Here's how the part is built. I have some questions about the finished solid (model axes, mm). A direction names the side the tool comes from. Coordinates: 2 decimals unless noted, no trailing zeros. Loops run counter-clockwise (first coordinate to the right, second up) from the corner with the lowest first, then second, coordinate; pieces in that order, holes last. Notation, with made-up numbers: (39.25, -2) -> (83.25, -2) arc R22 cw to (83.25, 24) -> close; hole circle Ø9 at (85, 62). An arc over 180 degrees is marked (long way). Answer as a JSON object with one key per item and string values. Group by question number.
1) I want a section at C-C (z = 0.9). Write out the boundary of the cut face in (x, y) (3 decimals).
2) I want a section at B-B (y = 8). Write out the boundary of the cut face in (x, z).
3) If we mould it in two halves opening along X, with no side actions, what happens to faces 6 (the flat face through (0, -33, 1)), 7 (the cylindrical face through (18.402, -32.257, 1.479)), 8 (the flat face through (0, -30, 1))? For each: +X half, -X half, draft (parallel to the pull), parting line (faces both ways), or undercut.
4) I want a section at D-D (x = 24.5). Write out the boundary of the cut face in (y, z) (3 decimals).
5) I want a section at A-A (x = 5.5). Write out the boundary of the cut face in (y, z) (3 decimals), then the cut area to 3 significant figures.
6) I need wall thicknesses on probe 1 along Y at (x, z) = (5.5, 1.8) (3 decimals); probe 2 along Y at (x, z) = (-0.5, 1.9); probe 3 along X at (y, z) = (13, 0.8). Which ranges of each line are inside material? Lowest first, please. Write a range as [from, to].
7) I'm going to push flat-ended pins straight in: pin 1 (1.5 mm diameter, centred on x = -15.5, z = 1.5, fed in from +Y); pin 2 (0.9 mm diameter, centred on x = 13.5, z = 1.5, fed in from -Y); pin 3 (1.5 mm diameter, centred on y = 19.5, z = 1, fed in from -X). Where does each tip first touch, or does it pass through?
8) Which directions (+Z, -Z, +X, -X, +Y, -Y) give clear straight access to the entire face, cutting with the end or side of a thin tool? Please do faces 1 (the flat face through (-14, -30, 1)), 2 (the flat face through (-16, -8.425, 1)), 3 (the cylindrical face through (-18.6, -32.2, 1.5)), 4 (the flat face through (0, 33, 1)), 5 (the flat face through (16, -27, 1)).
```python
from build123d import *

# Parameters (mm, degrees)
SALIENTE_EXTRUIR1_DEPTH = 3


with BuildPart() as part:
    # Croquis1 → Saliente-Extruir1 (new body)
    with BuildSketch(Plane.XY):
        with BuildLine():
            Line((-13, -33), (13, -33))
            ThreePointArc((13, -33), (18.477225575, -32.235384062), (23.535653753, -30))
            Line((23.535653753, -30), (4.502856857, -30))
            Line((4.502856857, -30), (4.502856857, -27))
            Line((4.502856857, -27), (27.282856857, -27))
            ThreePointArc((27.282856857, -27), (31.515630385, -20.561179235), (33, -13))
            Line((33, -13), (33, 13))
            ThreePointArc((33, 13), (27.142135624, 27.142135624), (13, 33))
            Line((13, 33), (-13, 33))
            ThreePointArc((-13, 33), (-27.142135624, 27.142135624), (-33, 13))
            Line((-33, 13), (-33, -13))
            ThreePointArc((-33, -13), (-31.515630385, -20.561179235), (-27.282856857, -27))
            Line((-27.282856857, -27), (-4.502856857, -27))
            Line((-4.502856857, -27), (-4.502856857, -30))
            Line((-4.502856857, -30), (-23.535653753, -30))
            ThreePointArc((-23.535653753, -30), (-18.477225575, -32.235384062), (-13, -33))
        make_face()
        Polygon((-30, -11.425), (-30, -8.425), (-1.5, -8.425), (-1.5, 30), (1.5, 30), (1.5, -8.425), (30, -8.425), (30, -11.425), (1.5, -11.425), (1.5, -30), (-1.5, -30), (-1.5, -11.425), align=None, mode=Mode.SUBTRACT)
    extrude(amount=SALIENTE_EXTRUIR1_DEPTH)


solid = part.part
```
Determined:
{
 "1": {"outline": "(-33, -13) arc R20 ccw to (-27.283, -27) -> (-4.503, -27) -> (-4.503, -30) -> (-23.536, -30) arc R20 ccw to (-13, -33) -> (13, -33) arc R20 ccw to (23.536, -30) -> (4.503, -30) -> (4.503, -27) -> (27.283, -27) arc R20 ccw to (33, -13) -> (33, 13) arc R20 ccw to (13, 33) -> (-13, 33) arc R20 ccw to (-33, 13) -> close; hole (-30, -11.425) -> (-1.5, -11.425) -> (-1.5, -30) -> (1.5, -30) -> (1.5, -11.425) -> (30, -11.425) -> (30, -8.425) -> (1.5, -8.425) -> (1.5, 30) -> (-1.5, 30) -> (-1.5, -8.425) -> (-30, -8.425) -> close"},
 "2": {"outline": "(-33, 0) -> (-1.5, 0) -> (-1.5, 3) -> (-33, 3) -> close; (1.5, 0) -> (33, 0) -> (33, 3) -> (1.5, 3) -> close"},
 "3": {"face 6": "draft", "face 7": "+X half", "face 8": "undercut"},
 "4": {"outline": "(-27, 0) -> (-11.425, 0) -> (-11.425, 3) -> (-27, 3) -> close; (-8.425, 0) -> (29.363, 0) -> (29.363, 3) -> (-8.425, 3) -> close"},
 "5": {"outline": "(-33, 0) -> (-30, 0) -> (-30, 3) -> (-33, 3) -> close; (-27, 0) -> (-11.425, 0) -> (-11.425, 3) -> (-27, 3) -> close; (-8.425, 0) -> (33, 0) -> (33, 3) -> (-8.425, 3) -> close", "area": "180 mm^2"},
 "6": {"probe 1": "[-33, -30], [-27, -11.425], [-8.425, 33]", "probe 2": "[-33, -30], [30, 33]", "probe 3": "[-33, -1.5], [1.5, 33]"},
 "7": {"pin 1": "y = 32.92", "pin 2": "y = -33", "pin 3": "x = -32.16"},
 "8": {"face 1": "+Z, -Z, -X", "face 2": "+Z, -Z", "face 3": "+Z, -Z, -X, -Y", "face 4": "+Z, -Z, +X, -X, +Y", "face 5": "+Z, -Z, +X"}
}
